from build123d import *

# Parameters (mm, degrees)
SKETCH1_W           = 140
SKETCH1_H           = 160
BOSS_EXTRUDE1_DEPTH = 3
SKETCH2_W           = 120
SKETCH2_H           = 120
SKETCH2_W_2         = 114
SKETCH2_H_2         = 114
BOSS_EXTRUDE2_DEPTH = 70
SKETCH4_W           = 120
SKETCH4_H           = 120
BOSS_EXTRUDE4_DEPTH = 3
SKETCH5_R           = 2.1
SKETCH5_W           = 39.9
SKETCH5_H           = 19.71
CUT_EXTRUDE2_DEPTH  = 3
SKETCH6_W           = 18.298163042
SKETCH6_H           = 17.309993256
CUT_EXTRUDE3_DEPTH  = 3
CUT_EXTRUDE8_DEPTH  = 5
SKETCH15_W          = 259.021634325
SKETCH15_H          = 180.269434884
BOSS_EXTRUDE5_DEPTH = 3
SKETCH18_R          = 1.6
CUT_EXTRUDE9_DEPTH  = 10
SKETCH19_W          = 12
SKETCH19_H          = 4.5
SKETCH19_H_2        = 8.4
SKETCH19_W_2        = 10.084057066
SKETCH19_H_3        = 7.362028533
CUT_EXTRUDE11_DEPTH = 5
SKETCH20_W          = 263.921538054
SKETCH20_H          = 19.630552878
SKETCH20_W_2        = 120
SKETCH20_H_2        = 3
CUT_EXTRUDE12_DEPTH = 233.259150239
SKETCH21_W          = 259.021634325
SKETCH21_H          = 40.269434884
CUT_EXTRUDE13_DEPTH = 209.619923406


with BuildPart() as part:
    # Sketch1 → Boss-Extrude1 (new body)
    with BuildSketch(Plane(origin=(0, 0, 0), x_dir=(1, 0, 0), z_dir=(0, 1, 0))):
        Rectangle(SKETCH1_W, SKETCH1_H)
    extrude(amount=BOSS_EXTRUDE1_DEPTH)

    # Sketch2 → Boss-Extrude2 (add)
    with BuildSketch(Plane(origin=(0, 3, 0), x_dir=(1, 0, 0), z_dir=(0, 1, 0))):
        Rectangle(SKETCH2_W, SKETCH2_H)
        Rectangle(SKETCH2_W_2, SKETCH2_H_2, mode=Mode.SUBTRACT)
    extrude(amount=BOSS_EXTRUDE2_DEPTH)

    # Sketch4 → Boss-Extrude4 (add)
    with BuildSketch(Plane(origin=(0, 73, 0), x_dir=(1, 0, 0), z_dir=(0, 1, 0))):
        Rectangle(SKETCH4_W, SKETCH4_H)
    extrude(amount=BOSS_EXTRUDE4_DEPTH)

    # Sketch5 → Cut-Extrude2 (cut)
    with BuildSketch(Plane(origin=(0, 76, 0), x_dir=(1, 0, 0), z_dir=(0, 1, 0))):
        with Locations(Location((34.39, -4.925, 0), (0, 0, 270))):
            Circle(SKETCH5_R)
        with Locations(Location((34.39, 4.925, 0), (0, 0, 270))):
            Circle(SKETCH5_R)
        with Locations(Location((-15.03, -4.925, 0), (0, 0, 270))):
            Circle(SKETCH5_R)
        with Locations(Location((-15.03, 4.925, 0), (0, 0, 270))):
            Circle(SKETCH5_R)
        with Locations((9.68, 0)):
            Rectangle(SKETCH5_W, SKETCH5_H)
    extrude(amount=-CUT_EXTRUDE2_DEPTH, mode=Mode.SUBTRACT)

    # Sketch6 → Cut-Extrude3 (cut)
    with BuildSketch(Plane(origin=(0, 76, 0), x_dir=(1, 0, 0), z_dir=(0, 1, 0))):
        Rectangle(SKETCH6_W, SKETCH6_H)
    extrude(amount=-CUT_EXTRUDE3_DEPTH, mode=Mode.SUBTRACT)

    # Sketch13 → Cut-Extrude8 (cut)
    with BuildSketch(Plane(origin=(0, 76, 0), x_dir=(1, 0, 0), z_dir=(0, 1, 0))):
        with BuildLine():
            ThreePointArc((-3.792582359, 49.728765052), (-53.491503795, -1.722579942), (-0.349490011, -49.609426409))
            ThreePointArc((-0.349490011, -49.609426409), (5.82592347, -42.51288634), (-1.270616599, -36.337472859))
            ThreePointArc((-1.270616599, -36.337472859), (-40.195607742, -1.261740085), (-3.792582359, 36.42488497))
            ThreePointArc((-3.792582359, 36.42488497), (2.859357682, 43.076825011), (-3.792582359, 49.728765052))
        make_face()
    extrude(amount=-CUT_EXTRUDE8_DEPTH, mode=Mode.SUBTRACT)

    # Sketch15 → Boss-Extrude5 (add)
    with BuildSketch(Plane(origin=(0, 3, 0), x_dir=(1, 0, 0), z_dir=(0, 1, 0))):
        with Locations((-39.510817163, -10.134717442)):
            Rectangle(SKETCH15_W, SKETCH15_H)
    extrude(amount=-BOSS_EXTRUDE5_DEPTH)

    # Sketch18 → Cut-Extrude9 (cut)
    with BuildSketch(Plane(origin=(0, 3, 0), x_dir=(1, 0, 0), z_dir=(0, 1, 0))):
        with Locations(Location((-55.452, -27.227420358, 0), (0, 0, 194.647469308))):
            Circle(SKETCH18_R)
        with Locations(Location((-55.452, 32.208579642, 0), (0, 0, 194.647469308))):
            Circle(SKETCH18_R)
        with Locations(Location((4.746, 32.208579642, 0), (0, 0, 270))):
            Circle(SKETCH18_R)
        with Locations(Location((4.746, -27.227420358, 0), (0, 0, 270))):
            Circle(SKETCH18_R)
    extrude(amount=-CUT_EXTRUDE9_DEPTH, mode=Mode.SUBTRACT)

    # Sketch19 → Cut-Extrude11 (cut)
    with BuildSketch(Plane.ZY.offset(60)):
        with Locations((12.367420358, 33)):
            Rectangle(SKETCH19_W, SKETCH19_H)
        with Locations((-11.259414931, 37.2)):
            Rectangle(SKETCH19_W, SKETCH19_H_2)
        with Locations((-28.606781654, 36.742945388)):
            Rectangle(SKETCH19_W_2, SKETCH19_H_3)
    extrude(amount=-CUT_EXTRUDE11_DEPTH, mode=Mode.SUBTRACT)

    # Sketch20 → Cut-Extrude12 (cut, through all)
    with BuildSketch(Plane.XY.offset(60)):
        with Locations((-37.060865298, -6.815276439)):
            Rectangle(SKETCH20_W, SKETCH20_H)
        with Locations((0, 74.5)):
            Rectangle(SKETCH20_W_2, SKETCH20_H_2)
    extrude(amount=-CUT_EXTRUDE12_DEPTH, mode=Mode.SUBTRACT)


with BuildPart() as cut_extrude12_piece_1:
    # of the separate pieces the step leaves, piece 1, a body of its own (cut_extrude12_pieces)
    add(part.part.solids().sort_by_distance((60, 73, 60))[0])


with BuildPart() as cut_extrude12_piece_2:
    # of the separate pieces the step leaves, piece 2, a body of its own (cut_extrude12_pieces)
    add(part.part.solids().sort_by_distance((90, 0, 60))[0])

    # Sketch21 → Cut-Extrude13 (cut, through all)
    with BuildSketch(Plane(origin=(0, 3, 0), x_dir=(1, 0, 0), z_dir=(0, 1, 0))):
        with Locations((-39.510817163, -80.134717442)):
            Rectangle(SKETCH21_W, SKETCH21_H)
    extrude(amount=-CUT_EXTRUDE13_DEPTH, mode=Mode.SUBTRACT)


solid = cut_extrude12_piece_1.part
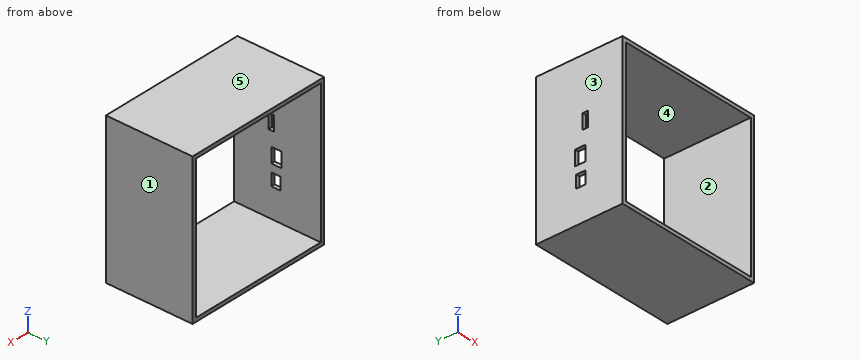
Model file for the job. Use its own axes, mm. Face numbers are marked on the shaded views. A direction names the side the tool comes from. Give positions to 0.01 mm unless a question says otherwise; leave off trailing zeros. Write each loop counter-clockwise with the first axis right and the second up, starting at its lowest first coordinate (ties: lowest second). Pieces come first, ordered by that corner, then holes. Notation, with made-up numbers: (81, 61) - (124, 61) arc R15 cw to (124, 87) - close; hole circle Ø8 at (21.25, 46.25). An arc over 180 degrees is marked (long way). Answer as CSV lines item,"result".
1. Two-plate mould, pull along X, no slides. Class the marked faces 3, 4 and 5: +X half, -X half, draft (parallel to the pull), parting line (faces both ways), or undercut.
Responses:
face 3,"-X half"
face 4,"undercut"
face 5,"draft"
2. Band-saw the part on A-A (z = 14.5). Write the cut outline in (x, y), and give its area (4 significant figures).
Responses:
outline,"(-60, 3) - (-57, 3) - (-57, 30.75) - (-60, 30.75) - close; (-60, 35.25) - (-57, 35.25) - (-57, 73) - (-60, 73) - close; (57, 3) - (60, 3) - (60, 73) - (57, 73) - close"
area,"406.5 mm2"
3. 3-axis set-ups, long thin cutter, end or side, ignore diameter. For the marked faces 1 and 2: which of +Z, -Z, +X, -X, +Y, -Y reach the whole face in a straight line?
Responses:
face 1,"+Z, -Z, +X, +Y, -Y"
face 2,"+Y, -Y"
4. Drill centre line: L1, parallel to Z at x = -44, y = 35.5. Where is it in solid material? Low to high. Write a range as [from, to].
Responses:
L1,"z = [-60, -57], [57, 60]"
5. Band-saw the part on D-D (y = 64.5). Write the cut outline in (x, z), and give its area (3 significant figures).
Responses:
outline,"(-60, -60) - (60, -60) - (60, 60) - (-60, 60) - close; hole (-57, -57) - (57, -57) - (57, 57) - (-57, 57) - close"
area,"1,400 mm2"
6. Band-saw the part on B-B (x = 36). Write the cut outline in (y, z).
Responses:
outline,"(3, -60) - (73, -60) - (73, -57) - (3, -57) - close; (3, 57) - (73, 57) - (73, 60) - (3, 60) - close"
7. Band-saw the part on C-C (z = -3). Write the cut outline in (x, y).
Responses:
outline,"(-60, 3) - (-57, 3) - (-57, 73) - (-60, 73) - close; (57, 3) - (60, 3) - (60, 73) - (57, 73) - close"
